from build123d import *

# Parameters (mm, degrees)
F0_R     = 0.748499
F0_R_2   = 1.073278
F0_W     = 4.846455
F0_H     = 1.625112
F1_DEPTH = 2.1


with BuildPart() as f1:
    # F0 (on Front) → F1 (new body)
    with BuildSketch(Plane.XZ):
        with BuildLine():
            ThreePointArc((-21.443578, 12.330635), (-21.622454, 9.776879), (-20.205865, 7.644522))
            Line((-20.205865, 7.644522), (-15.35941, 7.644522))
            ThreePointArc((-15.35941, 7.644522), (-13.844625, 10.276462), (-14.632234, 13.209269))
            ThreePointArc((-14.632234, 13.209269), (-15.513563, 14.050521), (-16.608446, 14.585011))
            ThreePointArc((-16.608446, 14.585011), (-18.11609, 14.748534), (-19.575115, 14.335043))
            ThreePointArc((-19.575115, 14.335043), (-20.687694, 13.49909), (-21.443578, 12.330635))
        make_face()
        with Locations((-19.575115, 11.795032)):
            Circle(F0_R, mode=Mode.SUBTRACT)
        with Locations((-15.838588, 11.580638)):
            Circle(F0_R_2, mode=Mode.SUBTRACT)
        Polygon((-15.35941, 6.01941), (-20.205865, 6.01941), (-22.600182, 6.01941), (-22.600182, 3.343472), (-22.600182, -5.8649), (-13.076994, -5.8649), (-13.076994, 3.343472), (-13.076994, 6.01941), align=None)
        with BuildLine():
            Line((-22.600182, 3.343472), (-22.600182, 6.01941))
            ThreePointArc((-22.600182, 6.01941), (-17.838588, 18.901843), (-13.076994, 6.01941))
            Line((-13.076994, 6.01941), (-13.076994, 3.343472))
            ThreePointArc((-13.076994, 3.343472), (-17.838588, 21.095032), (-22.600182, 3.343472))
        make_face()
        Polygon((-13.076994, -5.8649), (-22.600182, -5.8649), (-26.155973, -18.904968), (-20.811403, -18.904968), (-17.903329, -9.080392), (-14.995254, -18.904968), (-9.965071, -18.904968), align=None)
        with Locations((-17.782637, 6.831966)):
            Rectangle(F0_W, F0_H)
        with BuildLine():
            ThreePointArc((-19.575115, 14.335043), (-22.353082, 15.051527), (-21.443578, 12.330635))
            ThreePointArc((-21.443578, 12.330635), (-20.687694, 13.49909), (-19.575115, 14.335043))
        make_face()
        with BuildLine():
            ThreePointArc((-16.608446, 14.585011), (-15.513563, 14.050521), (-14.632234, 13.209269))
            ThreePointArc((-14.632234, 13.209269), (-14.074413, 16.117817), (-16.608446, 14.585011))
        make_face()
    extrude(amount=F1_DEPTH)


solid = f1.part
Can you work these out from the model? Positions are in its coordinate system, mm. A direction names the side the tool comes from. Give positions to 0.01 mm unless a question says otherwise; leave off trailing zeros. Loops run counter-clockwise (first coordinate to the right, second up) from the corner with the lowest first, then second, coordinate; pieces in that order, holes last. Notation, with made-up numbers: (-25.75, -24.75) - (-10.75, -24.75) arc R28 cw to (-10.75, 6.25) - close; hole circle Ø2 at (87.5, -5). An arc over 180 degrees is marked (long way). Answer as a JSON object with one key per item and string values.
Q1. If I drill on L1, parallel to Z at x = -22, y = -1.2; L2, parallel to X at y = -1, z = 11.5; L3, parallel to X at y = -1.45, z = -5, over which ranges is the centre line in solid material (lowest first)?
Geometry says:
{"L1": "-18.9 to 6.02, 12.54 to 15.34, 17.6 to 20.14", "L2": "-27.35 to -25.16, -21.69 to -20.26, -18.89 to -16.91, -14.77 to -13.87, -10.52 to -8.32", "L3": "-22.6 to -13.08"}
Q2. Imagine slicing it at A-A on z = -13.5. Write out the boundary of the cut face in (x, y).
Geometry says:
{"outline": "(-24.68, -2.1) - (-19.21, -2.1) - (-19.21, 0) - (-24.68, 0) - close; (-16.6, -2.1) - (-11.25, -2.1) - (-11.25, 0) - (-16.6, 0) - close"}
Q3. Imagine slicing it at B-B on x = -12. Write out the boundary of the cut face in (y, z).
Geometry says:
{"outline": "(-2.1, -18.9) - (0, -18.9) - (0, -10.38) - (-2.1, -10.38) - close; (-2.1, 4.07) - (0, 4.07) - (0, 7.16) - (-2.1, 7.16) - close; (-2.1, 16) - (0, 16) - (0, 19.09) - (-2.1, 19.09) - close"}
Q4. Imagine slicing it at D-D on z = 6.5. Write out the boundary of the cut face in (x, y), plus the area to 3 significant figures.
Geometry says:
{"outline": "(-25.88, -2.1) - (-23.11, -2.1) - (-23.11, 0) - (-25.88, 0) - close; (-20.21, -2.1) - (-15.36, -2.1) - (-15.36, 0) - (-20.21, 0) - close; (-12.57, -2.1) - (-9.79, -2.1) - (-9.79, 0) - (-12.57, 0) - close", "area": "21.8 mm²"}
Q5. Imagine slicing it at C-C on y = -0.85. Write out the boundary of the cut face in (x, z), plus the area to 3 significant figures.
Geometry says:
{"outline": "(-26.16, -18.9) - (-20.81, -18.9) - (-17.9, -9.08) - (-15, -18.9) - (-9.97, -18.9) - (-13.08, -5.86) - (-13.08, 3.34) arc R9.51 ccw (long way) to (-22.6, 3.34) - (-22.6, -5.86) - close; hole (-22.6, 6.02) - (-20.21, 6.02) - (-20.21, 7.64) arc R3.97 cw to (-21.44, 12.33) arc R1.63 cw (long way) to (-19.58, 14.34) arc R3.97 cw to (-16.61, 14.59) arc R1.62 cw (long way) to (-14.63, 13.21) arc R3.97 cw to (-15.36, 7.64) - (-15.36, 6.02) - (-13.08, 6.02) arc R7.32 ccw (long way) to start; hole circle Ø1.5 at (-19.58, 11.8); hole circle Ø2.15 at (-15.84, 11.58)", "area": "409 mm²"}
Q6. If we mould it in two halves opening along X, with no side actions, what happens to faces 1 (the cylindrical face through (-18.09, -1.04, 14.75)), 2 (the flat face through (-11.5, -1.04, -12.48)), 3 (the flat face through (-24, -1, -18.905))? For each: pulls with the +X half, pulls with the -X half, needs draft (parallel to the pull), parting line crosses it, or undercut.
Geometry says:
{"face 1": "undercut", "face 2": "pulls with the +X half", "face 3": "needs draft"}
Q7. Will these pins go through, and if not, where does the flat tip stop? P1, Ø1, axis at y = -1, z = 0.5, coming from the +X side; P2, Ø1, axis at y = -1, z = -1.5, coming from the -X side; P3, Ø0.6, axis at x = -21, y = -1, coming from the +Z side.
Geometry says:
{"P1": "x = -13.08", "P2": "x = -22.6", "P3": "z = 20.65"}
Q8. Which directions (+Z, -Z, +X, -X, +Y, -Y) give clear straight access to the entire face, cutting with the end or side of a thin tool? Please do faces 4 (the flat face through (-15.359, -1, 7)), 5 (the flat face through (-16.47, -1.04, -13.92)), 6 (the flat face through (-13.077, -1, -1)), 7 (the flat face through (-24.353, -1.035, -12.294)).
Geometry says:
{"face 4": "+Y, -Y", "face 5": "-Z, +Y, -Y", "face 6": "+X, +Y, -Y", "face 7": "-X, +Y, -Y"}
